Geometry check sheet. Reference: the model listing, model coordinates, mm. Face numbers are marked on the shaded views. A direction names the side the tool comes from. Coordinates: 2 decimals unless noted, no trailing zeros. Loops run counter-clockwise (first coordinate to the right, second up) from the corner with the lowest first, then second, coordinate; pieces in that order, holes last. Notation, with made-up numbers: M 16,33 L 39,33 A19 ccw 39,43 Z; hole C -36,31.25 d10. An arc over 180 degrees is marked long. One line per question, with ' | ' between items. Start each with the question number.
Autodesk Inventor part; units mm, degrees
ref_plane "YZ Plane" through (0, 0, 0) normal (1, 0, 0) x (0, 1, 0)
ref_plane "XZ Plane" through (0, 0, 0) normal (0, 1, 0) x (-1, 0, 0)
ref_plane "XY Plane" through (0, 0, 0) normal (0, 0, 1) x (1, 0, 0)
sketch "Sketch1" plane through (0, 0, 0) normal (0, 0, 1) x (1, 0, 0)
  line L0 (0, 0) -> (-11.15, 0)
  line L1 (-11.15, 0) -> (-11.15, 1)
  line L2 (-11.15, 1) -> (0, 1)
  line L3 (0, 1) -> (0, 2.5)
  line L4 (0, 2.5) -> (-11.15, 2.5)
  line L5 (-11.15, 2.5) -> (-11.15, 3.5)
  line L6 (-11.15, 3.5) -> (0, 3.5)
  line L7 (0, 3.5) -> (0, 5)
  line L8 (0, 5) -> (-11.15, 5)
  line L9 (-11.15, 5) -> (-11.15, 6)
  line L10 (-11.15, 6) -> (0, 6)
  line L11 (0, 6) -> (0, 7.5)
  line L12 (0, 7.5) -> (-11.15, 7.5)
  line L13 (-11.15, 7.5) -> (-11.15, 8.5)
  line L14 (-11.15, 8.5) -> (0, 8.5)
  line L15 (0, 8.5) -> (0, 10)
  line L16 (0, 10) -> (-11.15, 10)
  line L17 (-11.15, 10) -> (-11.15, 11)
  line L18 (-11.15, 11) -> (0, 11)
  line L19 (0, 11) -> (0, 12.5)
  line L20 (0, 12.5) -> (-11.15, 12.5)
  line L21 (-11.15, 12.5) -> (-11.15, 13.5)
  line L22 (-11.15, 13.5) -> (0, 13.5)
  line L23 (0, 13.5) -> (0, 15)
  line L24 (0, 15) -> (-11.15, 15)
  line L25 (-11.15, 15) -> (-11.15, 16)
  line L26 (-11.15, 16) -> (0, 16)
  line L27 (0, 16) -> (0, 17.5)
  line L28 (0, 17.5) -> (-11.15, 17.5)
  line L29 (-11.15, 17.5) -> (-11.15, 18.5)
  line L30 (-11.15, 18.5) -> (0, 18.5)
  line L31 (0, 18.5) -> (0, 20)
  line L32 (0, 20) -> (-11.15, 20)
  line L33 (-11.15, 20) -> (-11.15, 21)
  line L34 (-11.15, 21) -> (0, 21)
  line L35 (0, 21) -> (0, 22.5)
  line L36 (0, 22.5) -> (-11.15, 22.5)
  line L37 (-11.15, 22.5) -> (-11.15, 23.5)
  line L38 (-11.15, 23.5) -> (0, 23.5)
  line L39 (0, 23.5) -> (0, 25)
  line L40 (0, 25) -> (-11.15, 25)
  line L41 (-11.15, 25) -> (-11.15, 26)
  line L42 (-11.15, 26) -> (0, 26)
  line L43 (0, 26) -> (0, 27.5)
  line L44 (0, 27.5) -> (-8, 27.5)
  line L45 (-8, 27.5) -> (-8, 28.5)
  line L46 (-8, 28.5) -> (0, 28.5)
  line L47 (0, 28.5) -> (0, 27.5)
  line L48 (0, 26) -> (0, 25)
  line L49 (0, 23.5) -> (0, 22.5)
  line L50 (0, 21) -> (0, 20)
  line L51 (0, 18.5) -> (0, 17.5)
  line L52 (0, 16) -> (0, 15)
  line L53 (0, 13.5) -> (0, 12.5)
  line L54 (0, 11) -> (0, 10)
  line L55 (0, 8.5) -> (0, 7.5)
  line L56 (0, 6) -> (0, 5)
  line L57 (0, 3.5) -> (0, 2.5)
  line L58 (0, 1) -> (0, 0)
  dimension "d0" = 11.15
  dimension "d1" = 1
  dimension "d2" = 1.5
  dimension "d3" = 8
  dimension "d4" = 1
revolve "Fins" add sketch "Sketch1" angle 360 about axis through (0, 23.5, 0) along (0, 1, 0)
sketch "Sketch3" plane through (0, 0, 0) normal (1, 0, 0) x (0, 1, 0)
  line L0 (0, 0) -> (0, 7)
  line L1 (0, -11.15) -> (0, 11.15)
  line L2 (30, 5) -> (30, 8)
  line L3 (0, 7) -> (30, 5)
  line L4 (28.5, -8) -> (28.5, 8)
  line L5 (30, 8) -> (33, 8)
  line L6 (33, 8) -> (33, 6)
  line L7 (33, 6) -> (39, 6)
  line L8 (39, 6) -> (39, 8)
  line L9 (39, 8) -> (42.7, 8)
  line L10 (42.7, 8) -> (42.7, 0)
  line L11 (42.7, 0) -> (0, 0)
  dimension "d20" = 7
  dimension "d21" = 8
  dimension "d22" = 5
  dimension "d23" = 1.5
  dimension "d24" = 3
  dimension "d25" = 6
  dimension "d26" = 6
  dimension "d27" = 3.7
revolve "Body" add sketch "Sketch3" angle 360 about axis through (0, 42.7, 0) along (0, -1, 0)
sketch "Sketch4" plane through (0, 42.7, 0) normal (0, 1, 0) x (1, 0, 0)
  circle A0 centre (0, 0) radius 8
  circle A1 centre (0, 0) radius 4
  dimension "d29" = 8
extrude "CouplerHole" cut sketch "Sketch4" against normal blind 8 contours A1
sketch "Sketch5" plane through (0, 0, 0) normal (0, -1, 0) x (1, 0, 0)
  circle A0 centre (0, 0) radius 6.4333
  circle A1 centre (0, 0) radius 3.5
  dimension "d32" = 7
extrude "HeadBoltHole" cut sketch "Sketch5" against normal blind 14.8 contours A1
sketch "Sketch6" plane through (0, 14.8, 0) normal (0, -1, 0) x (1, 0, 0)
  circle A0 centre (0, 0) radius 3.5
  circle A1 centre (0, 0) radius 2.1
  dimension "d35" = 4.2
extrude "TubeHole" cut sketch "Sketch6" against normal up to surface (27.9 mm away) contours A1
properties part number "E3DV6HeatSink" material "Aluminum 6061"
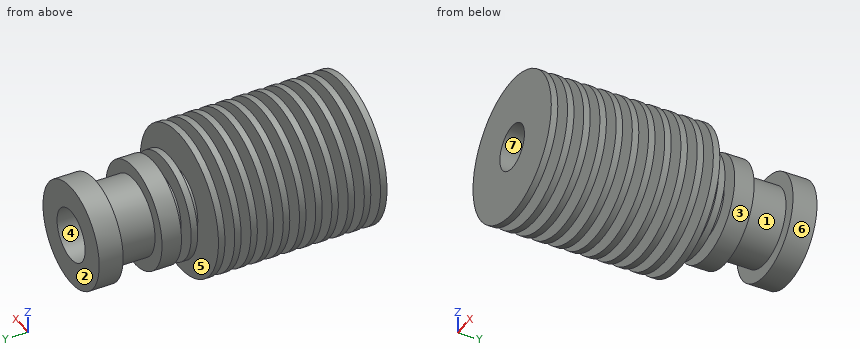
1. Tool access check on the marked faces 1, 2 and 3. Record the directions out of +Z, -Z, +X, -X, +Y, -Y that give a thin tool (end or side, any length) a straight path to the whole face; none if there is none.
2. Sectioned sample at C-C (x = -9). State how many separate pieces and enclosed holes the cut face has, and give its area (3 significant figures).
3. Sectioned sample at B-B (y = 32.5). Record the cut outline in (x, z).
4. Draft check along Z on the marked faces 4, 5, 6 and 7. Enter one of: +Z half, -Z half, draft (parallel to the pull), parting line (faces both ways), or undercut.
5. Sectioned sample at A-A (y = 9). Record the cut outline in (x, z), and give its area (3 significant figures).
6. Thickness scan on line 1 (Z direction, x = 0, y = 20.25); line 2 (Z direction, x = 0, y = 39.5); line 3 (Y direction, x = -3.5, z = -3.75). Record the ranges inside material, lowest first.
7. Depth check by flat-ended pin: pin 1 Ø6 at (x, y) = (-7.5, 8.5) entering from +Z; pin 2 Ø4 at (y, z) = (13.5, -7) entering from +X; pin 3 Ø12 at (y, z) = (13.5, 7) entering from -X. Enter the tip coordinate at first touch or a pass-through.
Result:
1) face 1: none | face 2: +Z, -Z, +X, -X, +Y | face 3: +Y
2) separate pieces: 11 | enclosed holes: 0 | area: 145 mm2
3) outline: C 0,0 d16; hole C 0,0 d4.2
4) face 4: undercut | face 5: draft | face 6: parting line | face 7: undercut
5) outline: C 0,0 d12.8; hole C 0,0 d7 | area: 90.2 mm2
6) line 1: z = -11.15 to -2.1, 2.1 to 11.15 | line 2: z = -8 to -4, 4 to 8 | line 3: y = 0 to 28.5, 30 to 42.7
7) pin 1: stops at z = 10.2 | pin 2: stops at x = 9.97 | pin 3: stops at x = -11.11
